Part model, mm, in its own coordinate system. A direction names the side the tool comes from. Coordinates: 2 decimals unless noted, no trailing zeros. Order: outer loops, then holes, each group sorted by start corner. A loop starts at its lowest first (then second) coordinate and runs counter-clockwise, first axis right, second up.
from build123d import *

# Parameters (mm, degrees)
SKETCH1_W           = 55
SKETCH1_H           = 14
BOSS_EXTRUDE1_DEPTH = 10
FILLET1_R           = 5
FILLET2_R           = 5
SKETCH2_R           = 4
CUT_EXTRUDE2_DEPTH  = 2.5
SKETCH3_R           = 2.1
CUT_EXTRUDE3_DEPTH  = 2
SKETCH4_R           = 3.95
CUT_EXTRUDE4_DEPTH  = 5
CUT_EXTRUDE5_REACH  = 64.926
SKETCH5_R           = 2
SKETCH7_R           = 2.1
CUT_EXTRUDE6_DEPTH  = 63.967570185
BOSS_EXTRUDE2_START = 2.5
SKETCH9_R           = 3.95
SKETCH9_R_2         = 2
BOSS_EXTRUDE2_DEPTH = 2.5
CUT_EXTRUDE7_START  = -3
SKETCH10_R          = 2
CUT_EXTRUDE7_DEPTH  = 3


with BuildPart() as part:
    # Sketch1 → Boss-Extrude1 (new body)
    with BuildSketch(Plane.XY):
        with Locations((-31.850618243, 13.301945946)):
            Rectangle(SKETCH1_W, SKETCH1_H)
    extrude(amount=BOSS_EXTRUDE1_DEPTH)

    # Fillet1
    fillet1_edges = [part.edges().sort_by_distance(p)[0] for p in [
        (-59.350618243, 20.301945946, 5),
    ]]
    fillet(fillet1_edges, radius=FILLET1_R)

    # Fillet2
    fillet2_edges = [part.edges().sort_by_distance(p)[0] for p in [
        (-4.350618243, 20.301945946, 5),
        (-4.350618243, 6.301945946, 5),
        (-59.350618243, 6.301945946, 5),
    ]]
    fillet(fillet2_edges, radius=FILLET2_R)

    # Sketch2 → Cut-Extrude2 (cut)
    with BuildSketch(Plane(origin=(0, 0, 0), x_dir=(-1, 0, 0), z_dir=(0, 0, -1))):
        with Locations((50.850618243, 13.301945946)):
            Circle(SKETCH2_R)
    extrude(amount=-CUT_EXTRUDE2_DEPTH, mode=Mode.SUBTRACT)

    # Sketch3 → Cut-Extrude3 (cut)
    with BuildSketch(Plane(origin=(0, 0, 2.5), x_dir=(-1, 0, 0), z_dir=(0, 0, -1))):
        with Locations((50.850618243, 13.301945946)):
            Circle(SKETCH3_R)
    extrude(amount=-CUT_EXTRUDE3_DEPTH, mode=Mode.SUBTRACT)

    # Sketch4 → Cut-Extrude4 (cut)
    with BuildSketch(Plane.XY.offset(10)):
        with Locations((-12.850618243, 13.301945946)):
            Circle(SKETCH4_R)
    extrude(amount=-CUT_EXTRUDE4_DEPTH, mode=Mode.SUBTRACT)

    # Sketch5 → Cut-Extrude5 (cut, up to next)
    with BuildSketch(Plane.XY.offset(5), mode=Mode.PRIVATE) as cut_extrude5_sk1:
        with Locations((-12.850618243, 13.301945946)):
            Circle(SKETCH5_R)
    cut_extrude5_tool1 = extrude(cut_extrude5_sk1.sketch, amount=-CUT_EXTRUDE5_REACH, mode=Mode.PRIVATE) & part.part
    add(cut_extrude5_tool1.solids().sort_by_distance((-12.850618, 13.301946, 5))[0], mode=Mode.SUBTRACT)

    # Sketch7 → Cut-Extrude6 (cut, through all)
    with BuildSketch(Plane(origin=(0, 0, 4.5), x_dir=(-1, 0, 0), z_dir=(0, 0, -1))):
        with Locations((50.850618243, 13.301945946)):
            Circle(SKETCH7_R)
    extrude(amount=-CUT_EXTRUDE6_DEPTH, mode=Mode.SUBTRACT)

    # Sketch9 → Boss-Extrude2 (add)
    with BuildSketch(Plane.XY.offset(5).offset(BOSS_EXTRUDE2_START)):
        with Locations((-12.850618243, 13.301945946)):
            Circle(SKETCH9_R)
        with Locations((-12.850618243, 13.301945946)):
            Circle(SKETCH9_R_2, mode=Mode.SUBTRACT)
    extrude(amount=-BOSS_EXTRUDE2_DEPTH)

    # Sketch10 → Cut-Extrude7 (cut)
    with BuildSketch(Plane(origin=(0, 0, 0), x_dir=(-1, 0, 0), z_dir=(0, 0, -1)).offset(CUT_EXTRUDE7_START)):
        Polygon((12.850618243, 17.34339783), (9.350618243, 15.322671888), (9.350618243, 11.281220004), (12.850618243, 9.260494062), (16.350618243, 11.281220004), (16.350618243, 15.322671888), align=None)
        with Locations(Location((12.850618243, 13.301945946, 0), (0, 0, 180))):
            Circle(SKETCH10_R, mode=Mode.SUBTRACT)
    extrude(amount=CUT_EXTRUDE7_DEPTH, mode=Mode.SUBTRACT)


solid = part.part
Q1. Pin check, flat tips, straight feed: pin 1 Ø2.5 at (x, y) = (-11.5, 13.5) entering from +Z; pin 2 Ø6.5 at (x, y) = (-12.85, 13.3) entering from -Z; pin 3 Ø5 at (x, y) = (-50.85, 13.3) entering from -Z. Stop position of each tip, or through.
Results list:
pin 1: stops at z = 7.5
pin 2: stops at z = 3
pin 3: stops at z = 2.5
Q2. Cut at B-B on z = 2. Write the cut outline in (x, y), and give its area (3 significant figures).
Results list:
outline: (-59.35, 11.3) arc R5 ccw to (-54.35, 6.3) - (-9.35, 6.3) arc R5 ccw to (-4.35, 11.3) - (-4.35, 15.3) arc R5 ccw to (-9.35, 20.3) - (-54.35, 20.3) arc R5 ccw to (-59.35, 15.3) - close; hole circle Ø8 at (-50.85, 13.3); hole (-16.35, 11.28) - (-12.85, 9.26) - (-9.35, 11.28) - (-9.35, 15.32) - (-12.85, 17.34) - (-16.35, 15.32) - close
area: 656 mm2
Q3. Mould opens along X. For faces 1 (the face through (-57.925, 18.798, 5.07)), 2 (the face through (-11, 12, 3)), 3 (the face through (-15.762, 15.972, 8.768)), 4 (the face through (-32, 13, 10)) say: pulls with the +X half, pulls with the -X half, needs draft (parallel to the pull), parting line crosses it, or undercut.
Results list:
face 1: pulls with the -X half
face 2: undercut
face 3: undercut
face 4: needs draft
Q4. Which spindle directions (+Z, -Z, +X, -X, +Y, -Y) get a long thin tool onto all of the face, cutting with end or side? Do faces 5 (the face through (-15, 14, 7.5)), 6 (the face through (-11.076, 10.285, 1.521)), 7 (the face through (-32, 20.302, 5)). Say none if no direction does.
Results list:
face 5: +Z
face 6: -Z
face 7: +Z, -Z, +X, -X, +Y
Q5. Cut at C-C on y = 16.75. Write the cut outline in (x, z), and give its area (3 significant figures).
Results list:
outline: (-59.14, 0) - (-52.88, 0) - (-52.88, 2.5) - (-48.82, 2.5) - (-48.82, 0) - (-13.88, 0) - (-13.88, 3) - (-11.82, 3) - (-11.82, 0) - (-4.56, 0) - (-4.56, 10) - (-10.92, 10) - (-10.92, 7.5) - (-14.78, 7.5) - (-14.78, 10) - (-59.14, 10) - close
area: 520 mm2
Q6. Cut at A-A on x = -51.5. Write the cut outline in (y, z), and give its area (3 significant figures).
Results list:
outline: (6.3, 0) - (9.36, 0) - (9.36, 2.5) - (11.3, 2.5) - (11.3, 10) - (6.3, 10) - close; (15.3, 2.5) - (17.25, 2.5) - (17.25, 0) - (20.3, 0) - (20.3, 10) - (15.3, 10) - close
area: 90.3 mm2
Q7. Wall check: line 1 along X through (y, z) = (13.5, 8.25); line 2 along X through (y, z) = (17, 1); line 3 along Z through (x, y) = (-10.5, 14). Give the ranges that are in metal, low to high.
Results list:
line 1: x = -59.35 to -52.94, -48.76 to -16.8, -8.91 to -4.35
line 2: x = -59.05 to -52.38, -49.33 to -13.45, -12.26 to -4.65
line 3: z = 3 to 7.5
Q8. Cut at D-D on x = -12. Write the cut outline in (y, z).
Results list:
outline: (6.3, 0) - (9.75, 0) - (9.75, 3) - (11.49, 3) - (11.49, 7.5) - (9.44, 7.5) - (9.44, 10) - (6.3, 10) - close; (15.11, 3) - (16.85, 3) - (16.85, 0) - (20.3, 0) - (20.3, 10) - (17.16, 10) - (17.16, 7.5) - (15.11, 7.5) - close
